```python
from build123d import *

# Parameters (mm, degrees)
SKETCH1_R           = 107
BOSS_EXTRUDE1_DEPTH = 6
SKETCH2_R           = 57
BOSS_EXTRUDE2_DEPTH = 1194
BOSS_EXTRUDE3_DEPTH = 195
CUT_EXTRUDE1_DEPTH  = 1210.772292624
CUT_EXTRUDE2_DEPTH  = 1210.772292624


with BuildPart() as part:
    # Sketch1 → Boss-Extrude1 (new body)
    with BuildSketch(Plane(origin=(0, 0, 0), x_dir=(1, 0, 0), z_dir=(0, 1, 0))):
        with Locations(Location((0, 0, 0), (0, 0, 270))):
            Circle(SKETCH1_R)
    extrude(amount=BOSS_EXTRUDE1_DEPTH)

    # Sketch2 → Boss-Extrude2 (add)
    with BuildSketch(Plane(origin=(0, 6, 0), x_dir=(1, 0, 0), z_dir=(0, 1, 0))):
        with Locations(Location((0, 0, 0), (0, 0, 270))):
            Circle(SKETCH2_R)
    extrude(amount=BOSS_EXTRUDE2_DEPTH)

    # Sketch3 → Boss-Extrude3 (add)
    with BuildSketch(Plane(origin=(0, 6, 0), x_dir=(1, 0, 0), z_dir=(0, 1, 0))):
        Polygon((-107, 0), (-107, -3), (-3, -3), (-3, -107), (3, -107), (3, -3), (107, -3), (107, 3), (3, 3), (3, 107), (0, 107), (-3, 107), (-3, 3), (-107, 3), align=None)
    extrude(amount=BOSS_EXTRUDE3_DEPTH)

    # Sketch4 → Cut-Extrude1 (cut, through all)
    with BuildSketch(Plane.XY.offset(3)):
        Polygon((-56.920997883, 201), (-107, 6), (-153.843462946, 6), (-153.843462946, 243.950118008), (-57, 243.950118008), align=None)
        Polygon((107, 6), (56.920997883, 201), (57, 243.950118008), (157.678532458, 243.950118008), (157.678532458, 6), align=None)
    extrude(amount=-CUT_EXTRUDE1_DEPTH, mode=Mode.SUBTRACT)

    # Sketch6 → Cut-Extrude2 (cut, through all)
    with BuildSketch(Plane.ZY.offset(3)):
        Polygon((-107, 6), (-56.920997883, 201), (-57, 265.799576447), (-234.352889602, 265.799576447), (-234.352889602, 6), align=None)
        Polygon((107, 6), (56.920997883, 201), (57, 265.799576447), (191.443205591, 265.799576447), (191.443205591, 6), align=None)
    extrude(amount=-CUT_EXTRUDE2_DEPTH, mode=Mode.SUBTRACT)


solid = part.part
```
Geometry: final body of the model. Coordinates: model frame, mm. A direction names the side the tool comes from. Round coordinates to 2 decimals unless told otherwise and drop trailing zeros. Order: outer loops, then holes, each group sorted by start corner. A loop starts at its lowest first (then second) coordinate and runs counter-clockwise, first axis right, second up. Notation, with made-up numbers: (58, 45) - (83, 45) arc R10 cw to (83, 62) - close; hole circle Ø1 at (-27.75, 38.25). An arc over 180 degrees is marked (long way). Write item = value, one per line. Start each with the question number.
Q1. Access query for faces 1 (the flat face through (76, 80, 3)), 2 (the flat face through (-54, 6, -56)), 3 (the flat face through (3, 80, -76)). Directions: +Z, -Z, +X, -X, +Y, -Y. A direction counts if a zero-diameter tool reaches every point of the face in a straight line with its end or side. Return the directions, or none.
Q2. Ray query, line 1 (Y direction, x = 76, z = -7.5); line 2 (X direction, y = 91.5, z = -66); line 3 (X direction, y = 782, z = 52.5). Return the intervals inside material, ascending. Write a range as from..to.
Q3. Cut plane C-C on y = 1083.5. Return the cut outline in (x, z), and give its area (3 significant figures).
Q4. Pin query (flat end, axial travel): pin 1 (1.5 mm diameter, centred on y = 576, z = 7, fed in from +X); pin 2 (3 mm diameter, centred on x = 8.5, y = 532.5, fed in from -Z); pin 3 (5 mm diameter, centred on y = 315, z = 50.5, fed in from -X); pin 4 (1 mm diameter, centred on x = -28, z = -46, fed in from -Y). Return the tip coordinate at first contact, or that it passes through.
Q5. Cut plane B-B on x = 33.5. Return the cut outline in (y, z).
Q6. Cut plane A-A on z = 26.5. Return the cut outline in (x, y).
Outcome:
q1.face_1 = +Z, +X, +Y
q1.face_2 = -Z, -X, +Y
q1.face_3 = -Z, +X, +Y
q2.line_1 = 0..6
q2.line_2 = -3..3
q2.line_3 = -22.2..22.2
q3.outline = circle Ø114 at (0, 0)
q3.area = 10,200 mm^2
q4.pin_1 = 56.66
q4.pin_2 = -56.57
q4.pin_3 = -30.74
q4.pin_4 = 0
q5.outline = (0, -101.62) - (6, -101.62) - (6, -46.12) - (1200, -46.12) - (1200, 46.12) - (6, 46.12) - (6, 101.62) - (0, 101.62) - close
q6.outline = (-103.67, 0) - (103.67, 0) - (103.67, 6) - (50.47, 6) - (50.47, 1200) - (-50.47, 1200) - (-50.47, 6) - (-103.67, 6) - close
